Verification items for this drawing (mm, ordinates from the low corner). A direction names the side the tool comes from. Coordinates: 2 decimals unless noted, no trailing zeros. Loops run counter-clockwise (first coordinate to the right, second up) from the corner with the lowest first, then second, coordinate; pieces in that order, holes last.
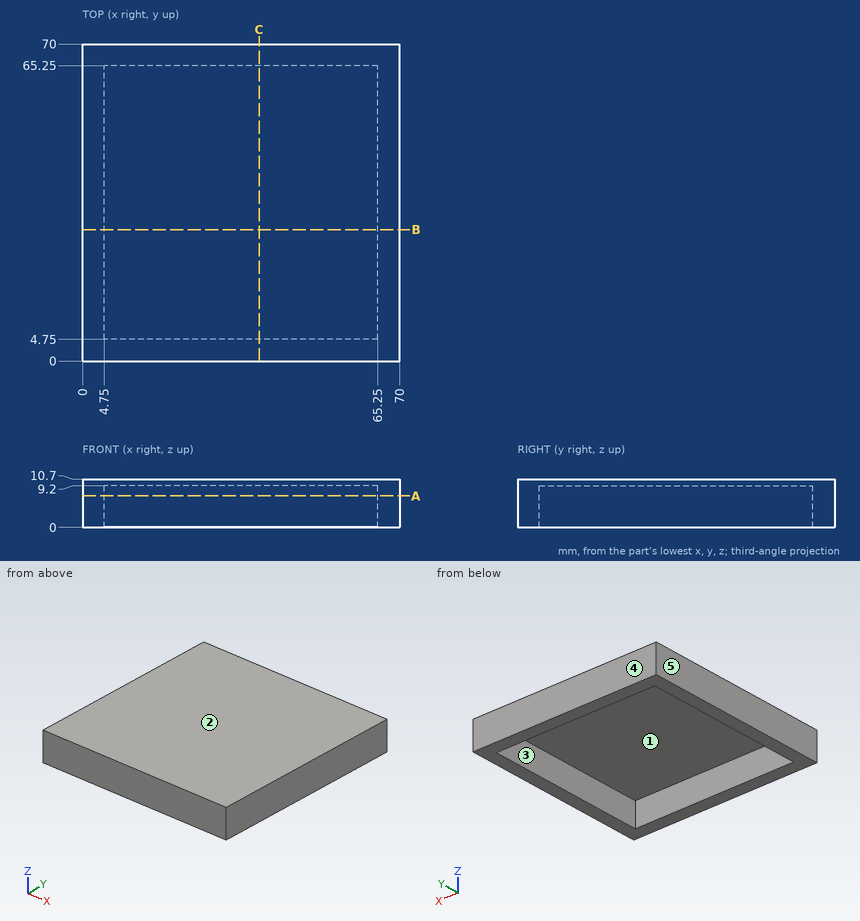
(1) Gauge pin test, flat end, axial feed: P1, Ø4.5, axis at x = 46, z = 3.5, coming from the -Y side. Record the tip position at first contact, or that the pin passes through.
(2) Section check B-B, the plane y = 29. Enter the section's corners in (x, z), plus the area to 3 significant figures.
(3) Scan lines: line 1 along X through (y, z) = (11, 6.5); line 2 along Z through (x, y) = (64.5, 18.5). Record each from-to range of solid material in increasing order.
(4) Set-up check for the marked faces 1 and 2: record each of +Z, -Z, +X, -X, +Y, -Y from which the full face is reachable in a straight line by a thin tool's end or side.
(5) Draft check along Y on the marked faces 3, 4 and 5. Enter one of: pulls with the +Y half, pulls with the -Y half, needs draft (parallel to the pull), parting line crosses it, or undercut.
(6) Section check A-A, the plane z = 7. Enter the section's corners in (x, y), plus the area to 3 significant figures.
Determined:
1. P1: stops at y = 0
2. outline: (0, 0) - (4.75, 0) - (4.75, 9.2) - (65.25, 9.2) - (65.25, 0) - (70, 0) - (70, 10.7) - (0, 10.7) - close
2. area: 192 mm2
3. line 1: x = 0 to 4.75, 65.25 to 70
3. line 2: z = 9.2 to 10.7
4. face 1: -Z
4. face 2: +Z, +X, -X, +Y, -Y
5. face 3: undercut
5. face 4: pulls with the +Y half
5. face 5: needs draft
6. outline: (0, 0) - (70, 0) - (70, 70) - (0, 70) - close; hole (4.75, 4.75) - (65.25, 4.75) - (65.25, 65.25) - (4.75, 65.25) - close
6. area: 1,240 mm2
